```python
from build123d import *

# Parameters (mm, degrees)
BOX_W         = 10.5
BOX_H         = 13.2
BOX_DEPTH     = 1.6
SKETCH_R      = 1
SKETCH_R_2    = 2
PAD_DEPTH     = 0.01
SKETCH001_R   = 1.5
SKETCH001_R_2 = 0.5
POCKET_DEPTH  = 1.611
SKETCH002_W   = 2.5
SKETCH002_H   = 2.5
PAD001_DEPTH  = 1
FILLET_R      = 0.5
FILLET001_R   = 0.3


with BuildPart() as part:
    # Box → Box (new body)
    with BuildSketch(Plane.XY):
        with Locations((5.25, 6.6)):
            Rectangle(BOX_W, BOX_H)
    extrude(amount=BOX_DEPTH)

    # Sketch → Pad (new body)
    with BuildSketch(Plane.XY.offset(1.6)):
        with Locations((1.44, 1.5)):
            Circle(SKETCH_R)
        with Locations((3.98, 1.5)):
            Circle(SKETCH_R)
        with Locations((6.52, 1.5)):
            Circle(SKETCH_R)
        with Locations((9.06, 1.5)):
            Circle(SKETCH_R)
        with Locations((7.75, 10.5)):
            Circle(SKETCH_R_2)
    extrude(amount=PAD_DEPTH)

    # Sketch001 → Pocket (cut, through all)
    with BuildSketch(Plane.XY.offset(1.61)):
        with Locations((7.75, 10.5)):
            Circle(SKETCH001_R)
        with Locations((1.44, 1.5)):
            Circle(SKETCH001_R_2)
        with Locations((3.98, 1.5)):
            Circle(SKETCH001_R_2)
        with Locations((6.52, 1.5)):
            Circle(SKETCH001_R_2)
        with Locations((9.06, 1.5)):
            Circle(SKETCH001_R_2)
    extrude(amount=-POCKET_DEPTH, mode=Mode.SUBTRACT)

    # Sketch002 → Pad001 (new body)
    with BuildSketch(Plane(origin=(0, 0, 0), x_dir=(1, 0, 0), z_dir=(0, 0, -1))):
        with Locations((2.95, -10.6)):
            Rectangle(SKETCH002_W, SKETCH002_H)
    extrude(amount=PAD001_DEPTH)

    # Fillet
    fillet_edges = [part.edges().sort_by_distance(p)[0] for p in [
        (4.2, 11.85, -0.5),
        (1.7, 11.85, -0.5),
        (1.7, 9.35, -0.5),
        (4.2, 9.35, -0.5),
    ]]
    fillet(fillet_edges, radius=FILLET_R)

    # Fillet001
    fillet001_edges = [part.edges().sort_by_distance(p)[0] for p in [
        (4.2, 10.6, -1),
        (2.95, 9.35, -1),
        (1.7, 10.6, -1),
        (2.95, 11.85, -1),
    ]]
    fillet(fillet001_edges, radius=FILLET001_R)


solid = part.part
```
The listing builds one solid part. Answer for the finished solid, in the listing's coordinates (mm). Coordinates: 2 decimals unless noted, no trailing zeros. Write each loop counter-clockwise with the first axis right and the second up, starting at its lowest first coordinate (ties: lowest second). Pieces come first, ordered by that corner, then holes. Notation, with made-up numbers: (27, -37) -> (51, -37) arc R37 ccw to (51, 0) -> close; hole circle Ø7 at (1.5, 41). An arc over 180 degrees is marked (long way). Write each question's results on one line, items separated by ' | '. Start each with the question number.
1) For a pull along X with two mould halves and no side action, classify faces 1 (the cylindrical face through (1.4, 2, 0.8)), 2 (the flat face through (0, 7, 1)), 3 (the flat face through (1, 1, 1.61)) as +X half, -X half, draft (parallel to the pull), parting line (faces both ways), or undercut.
2) Flat-ended cylindrical pins translate along their axes: pin 1 Ø3 at (x, y) = (6.5, 5.5) entering from +Z; pin 2 Ø0.6 at (x, z) = (3.5, -0.5) entering from -Y; pin 3 Ø0.6 at (x, z) = (2.5, -0.5) entering from +Y. Find the tip coordinate at first contact, or state that the pin passes through.
3) A cutting plane is placed at B-B (z = 0.75). Determine the outline of the cut face in (x, y), then the cut area to 3 significant figures.
4) Straight lines are drawn through the part: probe 1 along Y at (x, z) = (7.75, 0.7); probe 2 along Y at (x, z) = (1.44, 1); probe 3 along Z at (x, y) = (9.25, 7). For each, find the intervals that lie inside material, in ascending order.
5) A cutting plane is placed at D-D (x = 9.06). Count the separate pieces of the cut face and the enclosed holes in it, then the cut area to 3 significant figures.
Values follow:
1) face 1: undercut | face 2: -X half | face 3: draft
2) pin 1: z = 1.6 | pin 2: y = 9.35 | pin 3: y = 11.85
3) outline: (0, 0) -> (10.5, 0) -> (10.5, 13.2) -> (0, 13.2) -> close; hole circle Ø1 at (1.44, 1.5); hole circle Ø1 at (3.98, 1.5); hole circle Ø1 at (6.52, 1.5); hole circle Ø3 at (7.75, 10.5); hole circle Ø1 at (9.06, 1.5) | area: 128 mm²
4) probe 1: 0 to 9, 12 to 13.2 | probe 2: 0 to 1, 2 to 13.2 | probe 3: 0 to 1.6
5) separate pieces: 3 | enclosed holes: 0 | area: 17.2 mm²
